The drawing under review shows one solid part. Ordinate dimensions are in mm from its lowest x, y, z. A direction names the side the tool comes from. Coordinates: 2 decimals unless noted, no trailing zeros. Order: outer loops, then holes, each group sorted by start corner. A loop starts at its lowest first (then second) coordinate and runs counter-clockwise, first axis right, second up. Notation, with made-up numbers: (24.5, -13.75) -> (47.5, -13.75) arc R26 ccw to (47.5, 16.25) -> close; hole circle Ø5 at (64, -37.5). An arc over 180 degrees is marked (long way). Use one line per item in the form item = value.
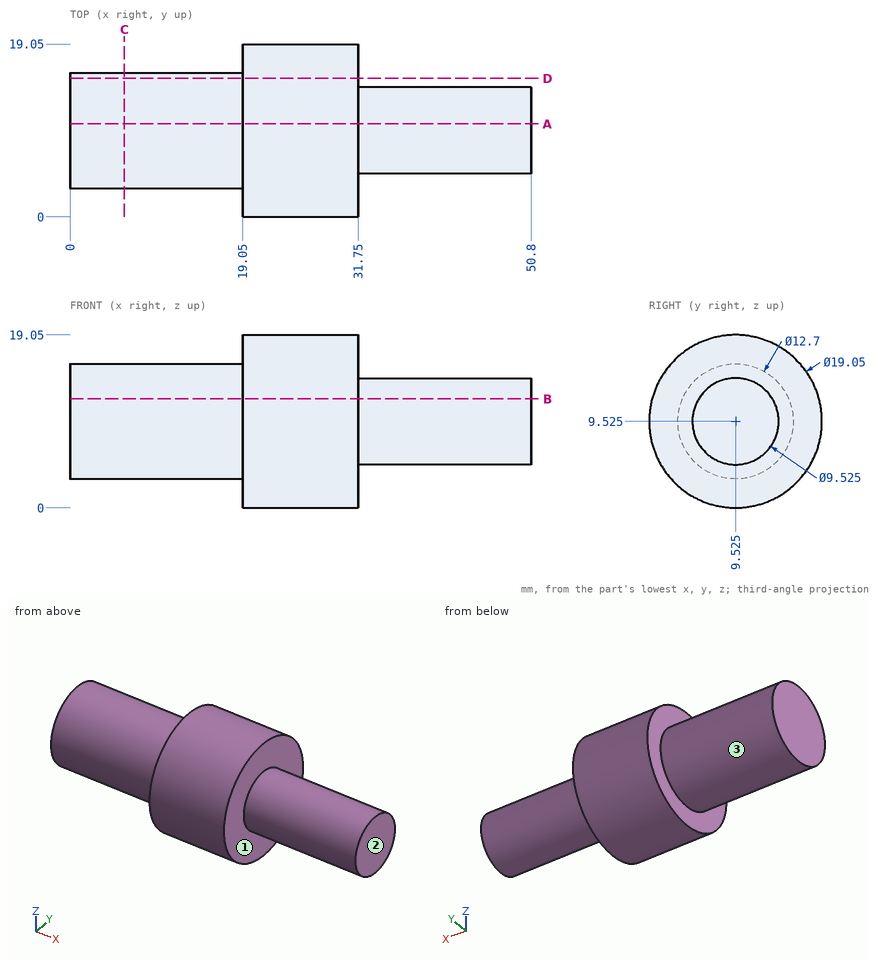
Item 1: We need section B-B (z = 12). Write out the cut boundary in (x, y).
Results found:
outline = (0, 3.68) -> (19.05, 3.68) -> (19.05, 0.33) -> (31.75, 0.33) -> (31.75, 5.46) -> (50.8, 5.46) -> (50.8, 13.59) -> (31.75, 13.59) -> (31.75, 18.72) -> (19.05, 18.72) -> (19.05, 15.37) -> (0, 15.37) -> close
Item 2: Clearance check with flat-ended pins moving along their axes: pin 1 (10 mm diameter, centred on x = 19, z = 14, fed in from +Y); pin 2 (6 mm diameter, centred on x = 14, z = 8.5, fed in from -Y) (3 decimals); pin 3 (8 mm diameter, centred on x = 15, y = 4.5, fed in from +Z); pin 4 (8 mm diameter, centred on x = 12, y = 12, fed in from +Z) (3 decimals). State where each tip first meets the part, or that it passes through.
Results found:
pin_1 = 19.05
pin_2 = 3.175
pin_3 = 15.79
pin_4 = 15.875
Item 3: We need section C-C (x = 6). Write out the cut boundary in (y, z) (3 decimals).
Results found:
outline = circle Ø12.7 at (9.525, 9.525)
Item 4: We need section A-A (y = 10.25). Write out the cut boundary in (x, z), plus the area to 3 significant figures.
Results found:
outline = (0, 3.22) -> (19.05, 3.22) -> (19.05, 0.03) -> (31.75, 0.03) -> (31.75, 4.82) -> (50.8, 4.82) -> (50.8, 14.23) -> (31.75, 14.23) -> (31.75, 19.02) -> (19.05, 19.02) -> (19.05, 15.83) -> (0, 15.83) -> close
area = 661 mm²
Item 5: We need section D-D (y = 15.25). Write out the cut boundary in (x, z), plus the area to 3 significant figures.
Results found:
outline = (0, 6.78) -> (19.05, 6.78) -> (19.05, 1.91) -> (31.75, 1.91) -> (31.75, 17.14) -> (19.05, 17.14) -> (19.05, 12.27) -> (0, 12.27) -> close
area = 298 mm²
Item 6: Tool access review of the marked faces 1, 2 and 3: name each direction out of +Z, -Z, +X, -X, +Y, -Y from which nothing blocks a thin tool from reaching the whole face with its end or side.
Results found:
face_1 = +X
face_2 = +Z, -Z, +X, +Y, -Y
face_3 = -X
Item 7: To check wall thickness, follow L1, parallel to X at y = 11.5, z = 16.25; L2, parallel to Y at x = 29.5, z = 3; L3, parallel to Z at x = 14, y = 7.75. State the ranges of each line that lie inside material, in increasing order. Write a range as from..to.
Results found:
L1 = 19.05..31.75
L2 = 2.59..16.46
L3 = 3.43..15.62
